Autodesk Fusion 360 part; units mm, degrees
sketch "Sketch9" plane through (0, 0, 0) normal (0, 0, 1) x (1, 0, 0)
  line L0 (3776.472, 1266.444) -> (3776.472, -304.8)
  line L1 (3776.472, 480.822) -> (2072.6401, 480.822)
  line L2 (3775.8634, 1264.9224) -> (3651.504, 954.024)
  line L3 (3651.504, 954.024) -> (3624.7105, 915.963)
  line L4 (2627.376, 883.92) -> (2761.488, 963.168)
  line L5 (2761.488, 963.168) -> (3394.4421, 1266.444)
  line L6 (3394.4421, 1266.444) -> (3775.8634, 1264.9224)
  line L7 (3775.8634, -303.2784) -> (3651.504, 7.62)
  line L8 (3651.504, 7.62) -> (3624.7105, 45.681)
  line L9 (2761.488, -1.524) -> (3394.4421, -304.8)
  line L10 (3394.4421, -304.8) -> (3775.8634, -303.2784)
  line L11 (2627.376, 77.724) -> (2761.488, -1.524)
  line L12 (2627.376, 883.92) -> (2627.376, 77.724)
  line L13 (3624.7105, 915.963) -> (3624.7105, 45.681)
  point P0 (3776.472, -304.8)
extrude "Extrude6" add sketch "Sketch9" along normal blind 213.36
sketch "Sketch10" plane through (0, 0, 0) normal (1, 0, 0) x (0, 1, 0)
  line L0 (1266.444, 220.98) -> (-304.8, 220.98) construction
  line L1 (480.822, 220.98) -> (480.822, -213.36)
  line L2 (908.185, 131.0434) -> (947.928, 149.352)
  line L3 (947.928, 149.352) -> (1225.8609, 152.5533)
  line L4 (1228.3549, 130.0128) -> (926.592, 112.776)
  line L5 (926.592, 112.776) -> (908.304, 118.872)
  arc A0 (1226.8338, 129.9259) -> (1225.8609, 152.5533) centre (1226.9491, 141.2655) ccw
  line L6 (908.185, 131.0434) -> (871.728, 131.0434)
  line L7 (871.728, 231.648) -> (1286.256, 231.648)
  line L8 (1286.256, 231.648) -> (1286.256, -12.192)
  line L9 (1286.256, -12.192) -> (871.728, -12.192)
  line L10 (871.728, 121.92) -> (908.304, 118.872)
  line L11 (53.459, 131.0434) -> (89.916, 131.0434)
  line L12 (53.459, 131.0434) -> (13.716, 149.352)
  line L13 (13.716, 149.352) -> (-264.2169, 152.5533)
  arc A1 (-264.2169, 152.5533) -> (-265.1898, 129.9259) centre (-265.3051, 141.2655) ccw
  line L14 (-266.7108, 130.0128) -> (35.052, 112.776)
  line L15 (35.052, 112.776) -> (53.34, 118.872)
  line L16 (89.916, 121.92) -> (53.34, 118.872)
  line L17 (-324.612, -12.192) -> (89.916, -12.192)
  line L18 (-324.612, 231.648) -> (-324.612, -12.192)
  line L19 (89.916, 231.648) -> (-324.612, 231.648)
  line L20 (871.728, 231.648) -> (89.916, 231.648)
  line L21 (871.728, -12.192) -> (89.916, -12.192)
  line L22 (871.728, 121.92) -> (89.916, 121.92)
  line L23 (871.728, 131.0434) -> (89.916, 131.0434)
extrude "Extrude7" cut sketch "Sketch10" along normal blind 4145.28
sketch "Sketch11" plane through (0, 0, 0) normal (0, 1, 0) x (1, 0, 0)
  line L0 (2590.8001, -213.36) -> (3810.0001, -213.36)
  line L1 (3810.0001, -213.36) -> (3810.0001, -30.48)
  line L2 (3810.0001, -30.48) -> (2590.8001, -30.48)
  line L3 (2590.8001, -30.48) -> (2590.8001, -213.36)
  line L4 (2753.8681, -128.1304) -> (2753.8681, -112.776)
  line L5 (2753.8681, -112.776) -> (3346.704, -91.44)
  line L6 (3346.704, -91.44) -> (3779.5201, -91.44)
  line L7 (3779.5201, -91.44) -> (3779.5201, -170.688)
  line L8 (2753.8681, -128.1304) -> (3493.008, -158.496)
  line L9 (3493.008, -158.496) -> (3779.5201, -170.688)
extrude "Extrude8" cut sketch "Sketch11" along normal mid plane 3108.96
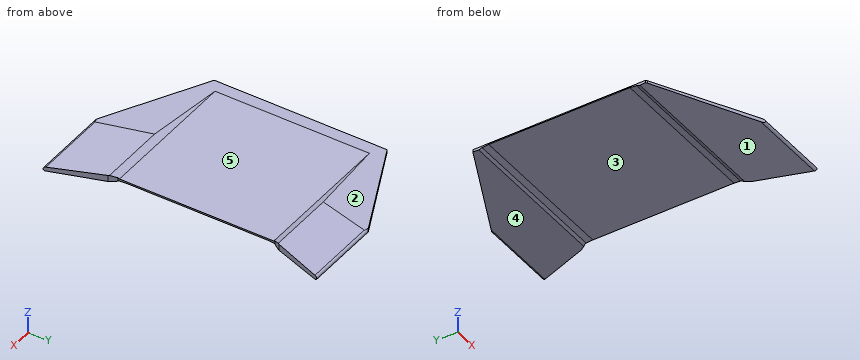
The model under review builds one solid part; all positions refer to its coordinate system, in mm. Face numbers are marked on the shaded views. A direction names the side the tool comes from. Round coordinates to 2 decimals unless told otherwise and drop trailing zeros. Write each loop counter-clockwise with the first axis right and the second up, starting at its lowest first coordinate (ties: lowest second). Pieces come first, ordered by that corner, then holes. Notation, with made-up numbers: (53, 74) - (96, 74) arc R11 cw to (96, 89) - close; hole circle Ø1 at (-5, -22.75). An arc over 180 degrees is marked (long way). Use one line per item in the form item = value.
Q1. Consider section C-C (x = 3220). State the section outline as (y, z) points (3 decimals), and give its area (3 significant figures).
Answer key:
outline = (-221.217, 127.414) - (35.052, 112.776) - (53.34, 118.872) - (89.916, 121.92) - (871.728, 121.92) - (908.304, 118.872) - (926.592, 112.776) - (1182.861, 127.414) - (1182.861, 147.28) - (943.431, 147.28) - (908.185, 131.043) - (53.459, 131.043) - (18.213, 147.28) - (-221.217, 147.28) - close
area = 22,400 mm2
Q2. Draft analysis for pull direction Y (two halves, no side actions). For the marked faces 1, 2 and 3, state which applies: +Y half, -Y half, draft (parallel to the pull), parting line (faces both ways), or undercut.
Answer key:
face_1 = -Y half
face_2 = draft
face_3 = undercut
Q3. For line 1 (Z direction, x = 3153, y = 758); line 2 (Y direction, x = 3669, z = 140); line 3 (Y direction, x = 3635, z = 142), list the stretches that pass through material, from the lowest coordinate up. Write a range as [from, to].
Answer key:
line_1 = [121.92, 131.04]
line_2 = [-276.57, -36.12], [997.76, 1238.22]
line_3 = [-276.62, 29.68], [931.97, 1238.27]
Q4. Consider section B-B (y = 694). State the section outline as (x, z) points, and give its area (3 significant figures).
Answer key:
outline = (2753.87, 121.92) - (3624.71, 121.92) - (3624.71, 131.04) - (2824.77, 131.04) - (2753.87, 128.13) - close
area = 7,840 mm2
Q5. Insertion check: pin 1 Ø1.5 at (x, z) = (3192.5, 133) entering from +Y; pin 2 Ø20 at (y, z) = (337, 129.5) entering from +X; pin 3 Ø5 at (x, y) = (3432.5, 323) entering from -Z. Each pin has a flat end and moves straight along its axis. Give the tip position at first contact, or say it passes through.
Answer key:
pin_1 = 1170.04
pin_2 = 3624.71
pin_3 = 121.92
Q6. Consider section A-A (z = 143). State the section outline as (x, y) points, and give its area (3 significant figures).
Answer key:
outline = (3115.81, -171.3) - (3335.4, -276.51) - (3765.16, -276.51) - (3651.5, 7.62) - (3637.51, 27.5) - (3115.81, 27.5) - close; (3115.81, 934.14) - (3637.51, 934.14) - (3651.5, 954.02) - (3765.16, 1238.16) - (3335.4, 1238.16) - (3115.81, 1132.94) - close
area = 335,000 mm2
Q7. Consider section D-D (y = 1116.5). State the section outline as (x, z) points, and give its area (3 significant figures).
Answer key:
outline = (3081.5, 123.62) - (3716.49, 123.62) - (3716.49, 151.29) - (3317.69, 151.29) - (3081.5, 141.59) - close
area = 16,400 mm2
Q8. Tool access review of the marked faces 4 and 5: name each direction out of +Z, -Z, +X, -X, +Y, -Y from which nothing blocks a thin tool from reaching the whole face with its end or side.
Answer key:
face_4 = -Z, +X, -X, +Y
face_5 = +Z, +X, -X
